Input: part model. Units: mm. Frame: model coordinates. Face numbers are marked on the shaded views. A direction names the side the tool comes from. Coordinates: 2 decimals unless noted, no trailing zeros. Order: outer loops, then holes, each group sorted by start corner. A loop starts at its lowest first (then second) coordinate and runs counter-clockwise, first axis right, second up.
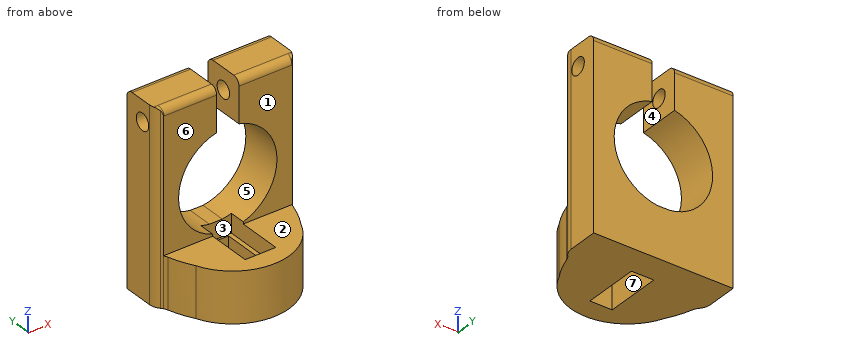
from build123d import *

# Parameters (mm, degrees)
SKETCH1_W               = 55
SKETCH1_H               = 40
BOSS_EXTRUDE1_DEPTH     = 18
SKETCH2_W               = 55
SKETCH2_H               = 15
BOSS_EXTRUDE2_DEPTH     = 50
CUT_EXTRUDE1_START      = -15
CUT_EXTRUDE1_DEPTH      = 15
SKETCH4_W               = 8
SKETCH4_H               = 40.233753348
CUT_EXTRUDE2_DEPTH      = 50
SKETCH6_R               = 3
CUT_EXTRUDE3_DEPTH      = 62
SKETCH7_W               = 8
SKETCH7_H               = 20
CUT_EXTRUDE4_DEPTH      = 18
CUT_EXTRUDE5_DEPTH      = 6
CUT_EXTRUDE5_DEPTH_BACK = 6
SKETCH8_W               = 11
SKETCH8_H               = 21.417406175
FILLET1_R               = 2.5
CUT_EXTRUDE6_DEPTH      = 67.335088131
CUT_EXTRUDE6_DEPTH_BACK = 67.335088131
CUT_EXTRUDE7_DEPTH      = 61
CUT_EXTRUDE8_DEPTH      = 39
FILLET2_R               = 20
CUT_EXTRUDE9_DEPTH      = 80.705724129
CUT_EXTRUDE9_DEPTH_BACK = 80.705724129
FILLET4_DEPTH           = 68
FILLET4_2_DEPTH         = 18
FILLET4_START           = -18
FILLET4_3_DEPTH         = 52
FILLET5_R               = 5


with BuildPart() as part:
    # Sketch1 → Boss-Extrude1 (new body)
    with BuildSketch(Plane.XY):
        with Locations((8.018292683, -5.274390244)):
            Rectangle(SKETCH1_W, SKETCH1_H)
    extrude(amount=BOSS_EXTRUDE1_DEPTH)

    # Sketch2 → Boss-Extrude2 (add)
    with BuildSketch(Plane.XY.offset(18)):
        with Locations((8.018292683, 7.225609756)):
            Rectangle(SKETCH2_W, SKETCH2_H)
    extrude(amount=BOSS_EXTRUDE2_DEPTH)

    # Cut-Extrude1: read off the stored shape, not the designer's step
    # Cut-Extrude1 outline → Cut-Extrude1 (cut)
    with BuildSketch(Plane(origin=(0, -0.274390244, 0), x_dir=(-1, 0, 0), z_dir=(0, -1, 0)).offset(CUT_EXTRUDE1_START)):
        with BuildLine():
            ThreePointArc((-10.314485184, -18), (-8.018292683, -53.15), (-5.722100182, -18))
            Line((-5.722100182, -18), (-10.314485184, -18))
        make_face()
    extrude(amount=CUT_EXTRUDE1_DEPTH, mode=Mode.SUBTRACT)

    # Sketch4 → Cut-Extrude2 (cut)
    with BuildSketch(Plane(origin=(0, -0.274390244, 0), x_dir=(-1, 0, 0), z_dir=(0, -1, 0))):
        with Locations((-8.018292683, -53.15)):
            Rectangle(SKETCH4_W, SKETCH4_H)
    extrude(amount=-CUT_EXTRUDE2_DEPTH, mode=Mode.SUBTRACT)

    # Sketch6 → Cut-Extrude3 (cut)
    with BuildSketch(Plane.ZY.offset(19.481707317)):
        with Locations(Location((60.5, 7.225609756, 0), (0, 0, 270))):
            Circle(SKETCH6_R)
    extrude(amount=-CUT_EXTRUDE3_DEPTH, mode=Mode.SUBTRACT)

    # Sketch7 → Cut-Extrude4 (cut)
    with BuildSketch(Plane(origin=(0, 0, 0), x_dir=(-1, 0, 0), z_dir=(0, 0, -1))):
        with Locations((-8.018292683, -5.274390244)):
            Rectangle(SKETCH7_W, SKETCH7_H)
    extrude(amount=-CUT_EXTRUDE4_DEPTH, mode=Mode.SUBTRACT)

    # Sketch8 → Cut-Extrude5 (cut, two sides: drawn at the far end of the back side and taken through both)
    with BuildSketch(Plane.XY.offset(18).offset(-CUT_EXTRUDE5_DEPTH_BACK)):
        with Locations((8.071503624, -5.248749455)):
            Rectangle(SKETCH8_W, SKETCH8_H)
    extrude(amount=CUT_EXTRUDE5_DEPTH + CUT_EXTRUDE5_DEPTH_BACK, mode=Mode.SUBTRACT)

    # Fillet1
    fillet1_edges = [part.edges().sort_by_distance(p)[0] for p in [
        (35.518292683, -12.774390244, 18),
        (-19.481707317, -12.774390244, 18),
        (-19.481707317, -0.274390244, 43),
        (35.518292683, -0.274390244, 43),
        (-7.731707317, -0.274390244, 68),
        (23.768292683, 14.725609756, 68),
        (8.018292683, -25.274390244, 18),
        (23.768292683, -0.274390244, 68),
        (-7.731707317, 14.725609756, 68),
        (-19.481707317, 14.725609756, 34),
        (35.518292683, 14.725609756, 34),
    ]]
    fillet(fillet1_edges, radius=FILLET1_R)

    # Sketch10 → Cut-Extrude6 (cut, two sides: drawn at the far end of the back side and taken through both)
    with BuildSketch(Plane.XY.offset(18).offset(-CUT_EXTRUDE6_DEPTH_BACK)):
        with BuildLine():
            ThreePointArc((-3.438146554, -22.774390244), (-11.4271438, -17.219826727), (-16.981707317, -9.230829481))
            Line((-16.981707317, -9.230829481), (-16.981707317, -22.774390244))
            Line((-16.981707317, -22.774390244), (-3.438146554, -22.774390244))
        make_face()
        with BuildLine():
            ThreePointArc((-16.981707317, -9.230829481), (-18.849438892, -3.637409944), (-19.481707317, 2.225609756))
            Line((-19.481707317, 2.225609756), (-19.481707317, -25.274390244))
            Line((-19.481707317, -25.274390244), (8.018292683, -25.274390244))
            ThreePointArc((8.018292683, -25.274390244), (2.155272983, -24.642121819), (-3.438146554, -22.774390244))
            Line((-3.438146554, -22.774390244), (-16.981707317, -22.774390244))
            Line((-16.981707317, -22.774390244), (-16.981707317, -9.230829481))
        make_face()
        with BuildLine():
            ThreePointArc((19.47473192, -22.774390244), (13.881312383, -24.642121819), (8.018292683, -25.274390244))
            Line((8.018292683, -25.274390244), (35.518292683, -25.274390244))
            Line((35.518292683, -25.274390244), (35.518292683, 2.225609756))
            ThreePointArc((35.518292683, 2.225609756), (34.886024258, -3.637409944), (33.018292683, -9.230829481))
            Line((33.018292683, -9.230829481), (33.018292683, -22.774390244))
            Line((33.018292683, -22.774390244), (19.47473192, -22.774390244))
        make_face()
        with BuildLine():
            ThreePointArc((33.018292683, -9.230829481), (27.463729166, -17.219826727), (19.47473192, -22.774390244))
            Line((19.47473192, -22.774390244), (33.018292683, -22.774390244))
            Line((33.018292683, -22.774390244), (33.018292683, -9.230829481))
        make_face()
    extrude(amount=CUT_EXTRUDE6_DEPTH + CUT_EXTRUDE6_DEPTH_BACK, mode=Mode.SUBTRACT)

    # Sketch11 → Cut-Extrude7 (cut)
    with BuildSketch(Plane(origin=(0, 14.725609756, 0), x_dir=(1, 0, 0), z_dir=(0, 1, 0))):
        Polygon((-16.981707317, -68), (-16.981707317, 0), (-29.965472326, 0), (-29.965472326, -73.975211298), (-16.981707317, -73.975211298), align=None)
    extrude(amount=-CUT_EXTRUDE7_DEPTH, mode=Mode.SUBTRACT)

    # Sketch12 → Cut-Extrude8 (cut)
    with BuildSketch(Plane(origin=(0, 14.725609756, 0), x_dir=(1, 0, 0), z_dir=(0, 1, 0))):
        Polygon((33.018292683, -34), (33.018292683, -69.603278632), (51.263623859, -69.603278632), (51.263623859, -68), (51.263623859, 5.657942166), (48.966322657, 5.657942166), (33.018292683, 5.657942166), align=None)
    extrude(amount=-CUT_EXTRUDE8_DEPTH, mode=Mode.SUBTRACT)

    # Fillet2
    fillet2_edges = [part.edges().sort_by_distance(p)[0] for p in [
        (-16.981707317, -9.230829481, 9),
        (33.018292683, -9.230829481, 9),
    ]]
    fillet(fillet2_edges, radius=FILLET2_R)

    # Sketch13 → Cut-Extrude9 (cut, two sides: drawn at the far end of the back side and taken through both)
    with BuildSketch(Plane(origin=(0, 0, 0), x_dir=(-1, 0, 0), z_dir=(0, 0, -1)).offset(-CUT_EXTRUDE9_DEPTH_BACK)):
        with BuildLine():
            Line((15.409844247, 2.637038383), (21.378631307, -1.925347001))
            Line((21.378631307, -1.925347001), (18.152736662, -25.695120221))
            Line((18.152736662, -25.695120221), (-4.693551269, -34.090790667))
            Line((-4.693551269, -34.090790667), (-38.816552793, -29.459816409))
            Line((-38.816552793, -29.459816409), (-43.750527307, -6.539564186))
            Line((-43.750527307, -6.539564186), (-31.534000974, 2.637038383))
            ThreePointArc((-31.534000974, 2.637038383), (-29.812131381, -4.006457809), (-26.853089861, -10.198787729))
            ThreePointArc((-26.853089861, -10.198787729), (-8.062078363, -22.773516814), (10.728933135, -10.198787729))
            ThreePointArc((10.728933135, -10.198787729), (13.687974655, -4.006457809), (15.409844247, 2.637038383))
        make_face()
    extrude(amount=CUT_EXTRUDE9_DEPTH + CUT_EXTRUDE9_DEPTH_BACK, mode=Mode.SUBTRACT)

    # Fillet4: read off the stored shape, not the designer's step
    # Fillet4 outline → Fillet4 (add)
    with BuildSketch(Plane.XY):
        with BuildLine():
            ThreePointArc((31.153095191, -0.274390244), (31.967368862, 0.746702465), (33.018292683, 1.52209337))
            Line((33.018292683, 1.52209337), (31.534000974, 2.637038383))
            ThreePointArc((31.534000974, 2.637038383), (31.270593615, 1.175225559), (30.946719887, -0.274390244))
            Line((30.946719887, -0.274390244), (31.153095191, -0.274390244))
        make_face()
        with BuildLine():
            ThreePointArc((-16.981707317, 1.435547188), (-15.921170685, 0.70393524), (-15.08279533, -0.274390244))
            Line((-15.08279533, -0.274390244), (-14.82256316, -0.274390244))
            ThreePointArc((-14.82256316, -0.274390244), (-15.146436888, 1.175225559), (-15.409844247, 2.637038383))
            Line((-15.409844247, 2.637038383), (-16.981707317, 1.435547188))
        make_face()
    extrude(amount=FILLET4_DEPTH)

    # Fillet4 2 outline → Fillet4 2 (add)
    with BuildSketch(Plane.XY):
        with BuildLine():
            ThreePointArc((30.624925491, -1.492895434), (30.848374458, -0.866028928), (31.153095191, -0.274390244))
            Line((31.153095191, -0.274390244), (30.946719887, -0.274390244))
            ThreePointArc((30.946719887, -0.274390244), (30.791189941, -0.885060274), (30.624925491, -1.492895434))
        make_face()
        with BuildLine():
            ThreePointArc((-15.08279533, -0.274390244), (-14.721255817, -0.92925432), (-14.461460233, -1.63072708))
            ThreePointArc((-14.461460233, -1.63072708), (-14.648665519, -0.954330135), (-14.82256316, -0.274390244))
            Line((-14.82256316, -0.274390244), (-15.08279533, -0.274390244))
        make_face()
    extrude(amount=FILLET4_2_DEPTH)

    # Fillet4 3 outline → Fillet4 3 (cut)
    with BuildSketch(Plane.YZ.offset(FILLET4_START)):
        with BuildLine():
            Line((-0.274390244, 68), (-0.274390244, 65.5))
            ThreePointArc((-0.274390244, 65.5), (0.457842803, 67.267766953), (2.225609756, 68))
            Line((2.225609756, 68), (-0.274390244, 68))
        make_face()
    extrude(amount=FILLET4_3_DEPTH, mode=Mode.SUBTRACT)

    # Fillet5
    # the kernel refuses this fillet: 5 mm, written as the material it takes off along each edge
    with BuildSketch(Plane(origin=(33.018292683, 1.52209337, 73.723867582), x_dir=(0, 1, 0), z_dir=(0, 0, -1))) as fillet5_piece_1:
        with BuildLine():
            CenterArc((2.329958397, -5), FILLET5_R, 90, 42.117992045)
            ThreePointArc((-1.023339511, -1.291173616), (-0.45812273, -0.688026327), (0, 0))
            Line((0, 0), (2.329958397, 0))
        make_face()
    extrude(amount=79.548763574, mode=Mode.SUBTRACT)
    with BuildSketch(Plane(origin=(-16.981707317, 1.435547188, -6.007429576), x_dir=(0, 1, 0), z_dir=(0, 0, 1))) as fillet5_piece_2:
        with BuildLine():
            CenterArc((2.40297183, -5), FILLET5_R, 90, 43.236885439)
            ThreePointArc((-1.022109439, -1.357361081), (-0.452973163, -0.72241666), (0, 0))
            Line((0, 0), (2.40297183, 0))
        make_face()
    extrude(amount=79.886736286, mode=Mode.SUBTRACT)


solid = part.part
Item 1: Ray query, probe 1 along X at (y, z) = (8, 56); probe 2 along X at (y, z) = (10.5, 35); probe 3 along Y at (x, z) = (19, 60). Return the intervals inside material, ascending.
Response values:
probe 1: x = -16.98 to 4.02, 12.02 to 33.02
probe 2: x = -16.98 to -9.62, 25.66 to 33.02
probe 3: y = -0.27 to 4.27, 10.18 to 14.73
Item 2: Cut plane B-B on z = 60.5. Return loops of the section in (x, y).
Response values:
outline: (-16.98, 3.84) arc R5 ccw to (-15.62, 0.41) arc R5 cw to (-15.08, -0.27) - (4.02, -0.27) - (4.02, 4.23) - (-16.98, 4.23) - close; (-16.98, 10.23) - (4.02, 10.23) - (4.02, 14.73) - (-16.98, 14.73) - close; (12.02, -0.27) - (31.15, -0.27) arc R5 cw to (31.73, 0.5) arc R5 ccw to (33.02, 3.85) - (33.02, 4.23) - (12.02, 4.23) - close; (12.02, 10.23) - (33.02, 10.23) - (33.02, 14.73) - (12.02, 14.73) - close
Item 3: Draft query along Z for the marked faces 1, 2 and 3. Return one class per face: pulls with the +Z half, pulls with the -Z half, needs draft (parallel to the pull), parting line crosses it, or undercut.
Response values:
face 1: needs draft
face 2: pulls with the +Z half
face 3: undercut
Item 4: Access query for the marked faces 4, 5, 6 and 7. Directions: +Z, -Z, +X, -X, +Y, -Y. A direction counts if a zero-diameter tool reaches every point of the face in a straight line with its end or side. Return the directions, or none.
Response values:
face 4: +Z, +Y, -Y
face 5: +Y, -Y
face 6: +Z, +X, -X, -Y
face 7: +Z, -Z
Item 5: Cut plane C-C on y = -12. Return loops of the section in (x, z).
Response values:
outline: (-9.88, 0) - (4.02, 0) - (4.02, 12) - (2.57, 12) - (2.57, 18) - (-9.88, 18) - close; (12.02, 0) - (26, 0) - (26, 18) - (13.57, 18) - (13.57, 12) - (12.02, 12) - close
Item 6: Cut plane D-D on z = 38.5. Return loops of the section in (x, y), then the cut area to 3 significant figures.
Response values:
outline: (-16.98, 3.84) arc R5 ccw to (-15.62, 0.41) arc R5 cw to (-15.08, -0.27) - (-9.37, -0.27) - (-9.37, 14.73) - (-16.98, 14.73) - close; (25.41, -0.27) - (31.15, -0.27) arc R5 cw to (31.73, 0.5) arc R5 ccw to (33.02, 3.85) - (33.02, 14.73) - (25.41, 14.73) - close
area: 223 mm2
Item 7: Cut plane A-A on x = 24. Return loops of the section in (y, z), then the cut area to 3 significant figures.
Response values:
outline: (-15.06, 0) - (14.73, 0) - (14.73, 28.01) - (-0.27, 28.01) - (-0.27, 18) - (-15.06, 18) - close; (-0.27, 42.99) - (14.73, 42.99) - (14.73, 65.5) arc R2.5 ccw to (12.23, 68) - (2.23, 68) arc R2.5 ccw to (-0.27, 65.5) - close; hole circle Ø6 at (7.23, 60.5)
area: 1,030 mm2
Item 8: Pin query (flat end, axial travel): pin 1 Ø2 at (y, z) = (-1, 15) entering from -X; pin 2 Ø4 at (x, z) = (7.5, 6.5) entering from -Y; pin 3 Ø2.5 at (x, y) = (7.5, 11) entering from +Z. Return the tip coordinate at first contact, or that it passes through.
Response values:
pin 1: stops at x = -15.28
pin 2: stops at y = -22.77
pin 3: stops at z = 18
